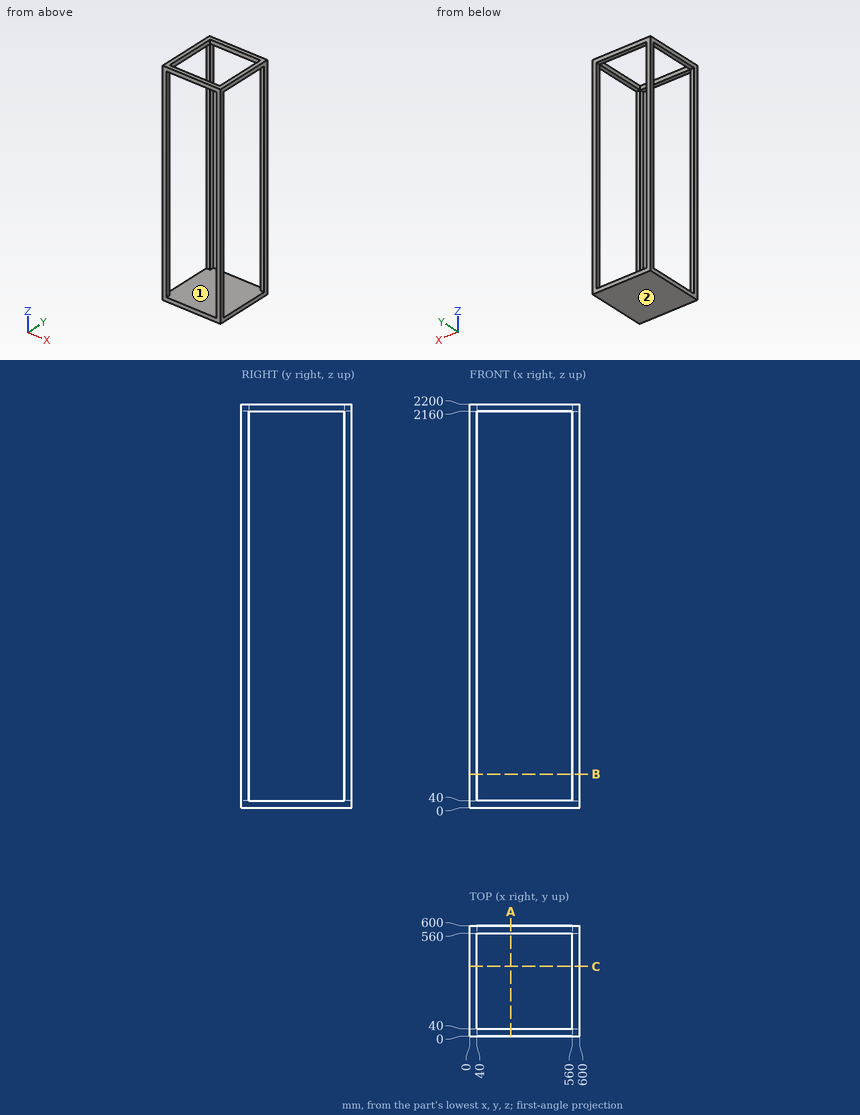
Here's the drawing with two shaded views (mm, measured from the low corner). I have some questions. Coordinates: 2 decimals unless noted, no trailing zeros. Write each loop counter-clockwise with the first axis right and the second up, starting at its lowest first coordinate (ties: lowest second). Pieces come first, ordered by that corner, then holes. Notation, with made-up numbers: M 0.25,31.25 L 45.25,31.25 A15 cw 45.25,40.25 Z; hole C 0,80 d11. An arc over 180 degrees is marked long. Write item = value, one per line. Start each with the question number.
Q1. If we section it at B-B, the plane z = 184: Write out the boundary of the cut face in (x, y), then the cut area to 3 significant figures.
Q2. If I drill on L1, parallel to Z at x = 232.5, y = 155.5, over which ranges is the centre line in solid material (lowest first)? Write a range as [from, to].
Q3. Thinking about a two-plate mould opening in Z: for the marked faces 1 and 2, which applies, released by +Z, released by -Z, zero draft, split by the parting line, or undercut?
Q4. I'm going to push a flat-ended pin straight in: pin 1 (10 mm diameter, centred on x = 383, y = 532.5, fed in from +Z). Where does the tip first touch, or does it pass through?
Q5. If we section it at A-A, the plane x = 225: Write out the boundary of the cut face in (y, z).
Check sheet entries:
q1.outline = M 0,0 L 40,0 L 40,40 L 0,40 Z; M 0,560 L 40,560 L 40,600 L 0,600 Z; M 560,0 L 600,0 L 600,40 L 560,40 Z; M 560,560 L 600,560 L 600,600 L 560,600 Z
q1.area = 6,400 mm²
q2.L1 = [0, 40]
q3.face_1 = undercut
q3.face_2 = released by -Z
q4.pin_1 = 40
q5.outline = M 0,0 L 600,0 L 600,40 L 0,40 Z; M 0,2160 L 40,2160 L 40,2200 L 0,2200 Z; M 560,2160 L 600,2160 L 600,2200 L 560,2200 Z
